from build123d import *

# Parameters (mm, degrees)
F1_DEPTH = 63.5
F2_DEPTH = 25.4
F3_DEPTH = 7.9375
F4_R     = 19.05
F0_W     = 20.32
F0_H     = 25.4


with BuildPart() as f1:
    # F0 (on Front) → F1 (new body, symmetric)
    with BuildSketch(Plane.XZ):
        Polygon((-59.020348, -9.525), (59.020348, -9.525), (59.020348, 9.525), (39.970348, 9.525), (-59.020348, 9.525), align=None)
    extrude(amount=F1_DEPTH, both=True)

    # F0 (on Front) → F2 (join, symmetric)
    with BuildSketch(Plane.XZ):
        with BuildLine():
            Line((39.970348, 9.525), (59.020348, 9.525))
            Line((59.020348, 9.525), (59.020348, 37.131319))
            ThreePointArc((59.020348, 37.131319), (60.435036, 44.631259), (64.484679, 51.100481))
            Line((64.484679, 51.100481), (90.776205, 51.100481))
            Line((90.776205, 51.100481), (90.776205, 70.150481))
            Line((90.776205, 70.150481), (57.678994, 70.150481))
            ThreePointArc((57.678994, 70.150481), (44.67694, 55.865387), (39.970348, 37.131319))
            Line((39.970348, 37.131319), (39.970348, 9.525))
        make_face()
        Polygon((90.776205, 73.233253), (90.776205, 70.150481), (90.776205, 51.100481), (90.776205, 47.833253), (111.096205, 47.833253), (111.096205, 73.233253), align=None)
    extrude(amount=F2_DEPTH, both=True)

    # F0 (on Front) → F3 (join, symmetric)
    with BuildSketch(Plane.XZ):
        with BuildLine():
            add(Edge.make_bspline(
                [(-59.020348, 9.525), (-47.986072, 47.833253), (-28.256564, 61.492361), (57.678994, 70.150481)],
                knots=[0, 0, 0, 0, 131.507358, 131.507358, 131.507358, 131.507358], degree=3))
            Line((-59.020348, 9.525), (39.970348, 9.525))
            Line((39.970348, 9.525), (39.970348, 37.131319))
            ThreePointArc((39.970348, 37.131319), (44.67694, 55.865387), (57.678994, 70.150481))
        make_face()
    extrude(amount=F3_DEPTH, both=True)

    # F4
    f4_edges = [f1.edges().sort_by_distance(p)[0] for p in [
        (59.020348, -63.5, 0),
        (-59.020348, -63.5, 0),
        (-59.020348, 63.5, 0),
        (59.020348, 63.5, 0),
    ]]
    fillet(f4_edges, radius=F4_R)

    # F0 (on Front) → F5 (revolve)
    with BuildSketch(Plane.XZ):
        with Locations((121.256205, 60.533253)):
            Rectangle(F0_W, F0_H)
    revolve(axis=Axis((111.096205, 0, 60.533253), (0, 0, 1)))


solid = f1.part
Can you work these out from the model? Positions are in its coordinate system, mm. A direction names the side the tool comes from. Give positions to 0.01 mm unless a question says otherwise; leave off trailing zeros. Loops run counter-clockwise (first coordinate to the right, second up) from the corner with the lowest first, then second, coordinate; pieces in that order, holes last. Notation, with made-up numbers: (68.25, -35.5) -> (78.25, -35.5) arc R18 ccw to (78.25, -19.5) -> close; hole circle Ø9 at (76, 46.5). An arc over 180 degrees is marked (long way). Use one line per item in the form item = value.
1) If we section it at A-A (y = 13): Please give me the cut outline in (x, z) (3 decimals), plus the area to 3 significant figures.
Answers:
outline = (-59.02, -9.525) -> (59.02, -9.525) -> (59.02, 37.131) arc R20.588 cw to (64.485, 51.1) -> (90.776, 51.1) -> (90.776, 47.833) -> (126.714, 47.833) -> (126.714, 73.233) -> (90.776, 73.233) -> (90.776, 70.15) -> (57.679, 70.15) arc R39.638 ccw to (39.97, 37.131) -> (39.97, 9.525) -> (-59.02, 9.525) -> close
area = 4,770 mm²
2) Will these pins go through, and if not, where does the flat tip stop? pin 1 (8 mm diameter, centred on x = 83.5, y = 12, fed in from -Z); pin 2 (5 mm diameter, centred on y = -28.5, z = 51, fed in from -X); pin 3 (18 mm diameter, centred on x = 25.5, z = 33.5, fed in from +Y); pin 4 (8 mm diameter, centred on x = 61, y = -10.5, fed in from -Z) (3 decimals).
Answers:
pin_1 = 51.1
pin_2 = through
pin_3 = 7.94
pin_4 = -9.525
3) If we section it at C-C (y = 51.5): Please give me the cut outline in (x, z) (3 decimals).
Answers:
outline = (-57.668, -9.525) -> (57.668, -9.525) -> (57.668, 9.525) -> (-57.668, 9.525) -> close
4) We'd pull the mould along X, two halves only. Please class faces 1 (the face through (131.41, -0.45, 60.71)), 2 (the face through (60.396, -0.356, 44.531)), 3 (the face through (1, -36, 9.525)): released by +X, released by -X, zero draft, split by the parting line, or undercut.
Answers:
face_1 = released by +X
face_2 = undercut
face_3 = zero draft
5) If we section it at B-B (y = 35.5): Please give me the cut outline in (x, z) (3 decimals), plus the area to 3 significant figures.
Answers:
outline = (-59.02, -9.525) -> (59.02, -9.525) -> (59.02, 9.525) -> (-59.02, 9.525) -> close
area = 2,250 mm²
6) I need wall thicknesses on line 1 along Y through (x, z) = (-4, 58); line 2 along Z through (x, y) = (-40, 28) (3 decimals); line 3 along Y through (x, z) = (55.5, 56.5). Which ranges of each line are inside material? Lowest first, please.
Answers:
line_1 = -7.94 to 7.94
line_2 = -9.525 to 9.525
line_3 = -25.4 to 25.4
7) For faces 4 (the face through (67, -25.4, 56)), 5 (the face through (74, 0, 70.15)), 6 (the face through (0, -7.938, 34)), 7 (the face through (39.97, 17, 24)), 8 (the face through (107, 0, 47.833)), which set-ups out of +Z, -Z, +X, -X, +Y, -Y let a thin tool reach every point of the face, with its end or its side?
Answers:
face_4 = +Z, +X, -X, -Y
face_5 = +Z, -X, +Y, -Y
face_6 = +Z, -X, -Y
face_7 = +Z, -X, +Y
face_8 = -Z, +X, +Y, -Y
